Can you work these out from the model? Positions are in its coordinate system, mm. Face numbers are marked on the shaded views. A direction names the side the tool comes from. Round coordinates to 2 decimals unless told otherwise and drop trailing zeros. Loops run counter-clockwise (first coordinate to the right, second up) from the corner with the lowest first, then second, coordinate; pieces in that order, holes last.
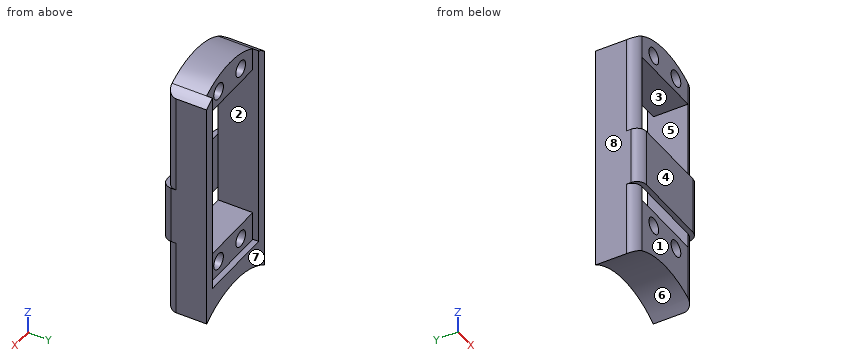
from build123d import *

# Parameters (mm, degrees)
BOSS_EXTRUDE1_DEPTH = 10.65022
SKETCH3_W           = 20.32
SKETCH3_H           = 7.62
CUT_EXTRUDE1_DEPTH  = 1.5494
SKETCH4_R           = 2.12598
CUT_EXTRUDE2_DEPTH  = 19.3294
SKETCH5_R           = 2.12598
BOSS_EXTRUDE2_DEPTH = 9.10082
SKETCH6_W           = 25.4
SKETCH6_H           = 1.27
BOSS_EXTRUDE3_DEPTH = 15.24
FILLET1_R           = 2.54
FILLET2_R           = 2.54


with BuildPart() as part:
    # Sketch2 → Boss-Extrude1 (new body)
    with BuildSketch(Plane(origin=(0, 0, 0), x_dir=(1, 0, 0), z_dir=(0, 1, 0))):
        with BuildLine():
            Line((-12.7, 45.261013597), (-12.7, -15.927319066))
            ThreePointArc((-12.7, -15.927319066), (-11.462644476, -16.839752797), (-10.16, -17.656270632))
            Line((-10.16, -17.656270632), (-10.16, 29.21))
            Line((-10.16, 29.21), (10.16, 29.21))
            Line((10.16, 29.21), (10.16, -17.656270632))
            ThreePointArc((10.16, -17.656270632), (11.462644476, -16.839752797), (12.7, -15.927319066))
            Line((12.7, -15.927319066), (12.7, 45.261013597))
            ThreePointArc((12.7, 45.261013597), (0, 41.275), (-12.7, 45.261013597))
        make_face()
    extrude(amount=-BOSS_EXTRUDE1_DEPTH)

    # Sketch3 → Cut-Extrude1 (cut)
    with BuildSketch(Plane(origin=(0, 0, 0), x_dir=(1, 0, 0), z_dir=(0, 1, 0))):
        with Locations((0, 33.02)):
            Rectangle(SKETCH3_W, SKETCH3_H)
    extrude(amount=-CUT_EXTRUDE1_DEPTH, mode=Mode.SUBTRACT)

    # Sketch4 → Cut-Extrude2 (cut)
    with BuildSketch(Plane(origin=(0, -1.5494, 0), x_dir=(1, 0, 0), z_dir=(0, 1, 0))):
        with Locations(Location((-4.87426, 33.12414, 0), (0, 0, 270))):
            Circle(SKETCH4_R)
        with Locations(Location((4.87426, 33.12414, 0), (0, 0, 270))):
            Circle(SKETCH4_R)
    extrude(amount=-CUT_EXTRUDE2_DEPTH, mode=Mode.SUBTRACT)

    # Sketch5 → Boss-Extrude2 (add)
    with BuildSketch(Plane(origin=(0, -1.5494, 0), x_dir=(1, 0, 0), z_dir=(0, 1, 0))):
        with BuildLine():
            Line((10.16, -11.684), (-10.16, -11.684))
            Line((-10.16, -11.684), (-10.16, -17.656270632))
            ThreePointArc((-10.16, -17.656270632), (0, -20.3708), (10.16, -17.656270632))
            Line((10.16, -17.656270632), (10.16, -11.684))
        make_face()
        with Locations(Location((4.87426, -15.47622, 0), (0, 0, 270))):
            Circle(SKETCH5_R, mode=Mode.SUBTRACT)
        with Locations(Location((-4.87426, -15.47622, 0), (0, 0, 270))):
            Circle(SKETCH5_R, mode=Mode.SUBTRACT)
    extrude(amount=-BOSS_EXTRUDE2_DEPTH)

    # Sketch6 → Boss-Extrude3 (add)
    with BuildSketch(Plane.XY.offset(-10.16)):
        with Locations((0, -11.28522)):
            Rectangle(SKETCH6_W, SKETCH6_H)
    extrude(amount=-BOSS_EXTRUDE3_DEPTH)

    # Fillet1
    fillet1_edges = [part.edges().sort_by_distance(p)[0] for p in [
        (12.7, -10.65022, 2.883659533),
        (-12.7, -10.65022, 2.883659533),
        (-12.7, -10.65022, -35.330506799),
        (12.7, -10.65022, -35.330506799),
    ]]
    fillet(fillet1_edges, radius=FILLET1_R - 0.0001)  # a hair under: the kernel refuses the full size

    # Fillet2
    fillet2_edges = [part.edges().sort_by_distance(p)[0] for p in [
        (-12.7, -11.92022, -17.78),
        (12.7, -11.92022, -17.78),
    ]]
    fillet(fillet2_edges, radius=FILLET2_R)


solid = part.part
(1) Will these pins go through, and if not, where does the flat tip stop? P1, Ø7.5, axis at x = -3.5, z = -15.5, coming from the +Y side; P2, Ø7, axis at x = 4.87, z = 15.48, coming from the -Y side; P3, Ø8.5, axis at x = 1, z = -32.5, coming from the +Y side.
Worked answers:
P1: stops at y = -10.65
P2: stops at y = -10.65
P3: stops at y = -1.55
(2) If we section it at B-B, the plane x = -9.5: List the corners of the cut face in (y, z) for me.
Worked answers:
outline: (-11.92, -25.4) - (-10.65, -25.4) - (-10.65, -10.16) - (-11.92, -10.16) - close; (-10.65, -43.41) - (0, -43.41) - (0, -36.83) - (-1.55, -36.83) - (-1.55, -29.21) - (-10.65, -29.21) - close; (-10.65, 11.68) - (-1.55, 11.68) - (-1.55, 18.02) - (-10.65, 18.02) - close
(3) For the marked faces 1, 2, 3 and 4, which set-ups out of +Z, -Z, +X, -X, +Y, -Y let a thin tool reach every point of the face, with its end or its side?
Worked answers:
face 1: -Z, +X, -X, -Y
face 2: +Y
face 3: +Y, -Y
face 4: +Z, -Z, +X, -X, -Y
(4) If we section it at D-D, the plane y = -4: List the corners of the cut face in (x, z) for me (3 decimals), then the cut area to 3 significant figures.
Worked answers:
outline: (-12.7, -45.261) arc R22.225 cw to (12.7, -45.261) - (12.7, 15.927) arc R20.371 ccw to (-12.7, 15.927) - close; hole (-10.16, -29.21) - (10.16, -29.21) - (10.16, 11.684) - (-10.16, 11.684) - close; hole circle Ø4.252 at (-4.874, -33.124); hole circle Ø4.252 at (-4.874, 15.476); hole circle Ø4.252 at (4.874, -33.124); hole circle Ø4.252 at (4.874, 15.476)
area: 675 mm2
(5) If we mould it in two halves opening along X, with no side actions, what happens to the marked faces 5, 6, 7 and 8? For each: released by +X, released by -X, zero draft, split by the parting line, or undercut.
Worked answers:
face 5: undercut
face 6: undercut
face 7: zero draft
face 8: released by -X
(6) If we section it at C-C, the plane z = -34.5: List the corners of the cut face in (x, y) for me (3 decimals), then the cut area to 3 significant figures.
Worked answers:
outline: (-12.7, -8.11) arc R2.54 ccw to (-10.16, -10.65) - (-6.495, -10.65) - (-6.495, -1.549) - (-10.16, -1.549) - (-10.16, 0) - (-12.7, 0) - close; (-3.254, -10.65) - (3.254, -10.65) - (3.254, -1.549) - (-3.254, -1.549) - close; (6.495, -10.65) - (10.16, -10.65) arc R2.54 ccw to (12.7, -8.11) - (12.7, 0) - (10.16, 0) - (10.16, -1.549) - (6.495, -1.549) - close
area: 177 mm2
(7) If I drill on line 1 (X direction, y = -5, z = -16); line 2 (Z direction, x = -3.5, y = -7.5); line 3 (Z direction, x = 5, y = -3), over which ranges is the centre line in solid material (lowest first)?
Worked answers:
line 1: x = -12.7 to -10.16, 10.16 to 12.7
line 2: z = -41.55 to -34.75, -31.5 to -29.21, 11.68 to 13.85, 17.1 to 20.07
line 3: z = -41.84 to -35.25, -31 to -29.21, 11.68 to 13.35, 17.6 to 19.75
